For this review, take the finished solid that the model builds, in its own axes (mm). A direction names the side the tool comes from. Coordinates: 2 decimals unless noted, no trailing zeros. Write each loop counter-clockwise with the first axis right and the second up, starting at its lowest first coordinate (ties: lowest second). Pieces come first, ordered by that corner, then holes. Notation, with made-up numbers: M 0,76.25 L 5,76.25 A15 ccw 5,94.25 Z; hole C 18.5,22.5 d2. An arc over 180 degrees is marked long. One line per question, with ' | ' between items.
from build123d import *

# Parameters (mm, degrees)
F0_R     = 11.5
F0_R_2   = 8.5
F1_DEPTH = 3
F0_R_3   = 6
F2_DEPTH = 14
F3_SIZE  = 1


with BuildPart() as f1:
    # F0 (on Front) → F1 (new body)
    with BuildSketch(Plane.XZ):
        Circle(F0_R)
        Circle(F0_R_2, mode=Mode.SUBTRACT)
    extrude(amount=F1_DEPTH)

    # F0 (on Front) → F2 (join)
    with BuildSketch(Plane.XZ):
        Circle(F0_R_2)
        Circle(F0_R_3, mode=Mode.SUBTRACT)
    extrude(amount=F2_DEPTH)

    # F3
    f3_edges = [f1.edges().sort_by_distance(p)[0] for p in [
        (-8.5, -14, 0),
        (-11.5, 0, 0),
    ]]
    chamfer(f3_edges, length=F3_SIZE)


solid = f1.part
1) We need section B-B on x = 0. State the section outline as (y, z) points, then the cut area to 3 significant figures.
Responses:
outline: M -14,-7.5 L -13,-8.5 L -3,-8.5 L -3,-11.5 L -1,-11.5 L 0,-10.5 L 0,-6 L -14,-6 Z; M -14,6 L 0,6 L 0,10.5 L -1,11.5 L -3,11.5 L -3,8.5 L -13,8.5 L -14,7.5 Z | area: 86.0 mm^2
2) Machinability: for faces 1 (the flat face through (2, -14, 6)), 2 (the cylindrical face through (4.57, -7.93, 7.167)), which of the approach directions +Z, -Z, +X, -X, +Y, -Y give a long, thin tool a straight path to every point of the face, cutting with its end or side? Answer none if there is none.
Responses:
face 1: +Z, -Z, +X, -X, -Y | face 2: -Y
3) Insertion check: pin 1 Ø8 at (x, y) = (-1, -2) entering from +Z; pin 2 Ø5 at (x, y) = (2, -5) entering from -Z; pin 3 Ø1 at (x, y) = (2.5, -6.5) entering from -Z; pin 4 Ø2 at (x, y) = (0, -8.5) entering from +Z. Each pin has a flat end and moves straight along its axis. Give the tip position at first contact, or say it passes through.
Responses:
pin 1: z = 11.5 | pin 2: z = -11.49 | pin 3: z = -8.26 | pin 4: z = 8.5
4) The part is to be moulded in two halves that separate along X. For faces 3 (the cylindrical face through (-6, -7, 0)), 4 (the cylindrical face through (-1.5, -2, 11.4)), 5 (the flat face through (5, 0, -5)), say which applies: +X half, -X half, draft (parallel to the pull), parting line (faces both ways), or undercut.
Responses:
face 3: undercut | face 4: parting line | face 5: draft
5) We need section A-A on z = 0. State the section outline as (x, y) points.
Responses:
outline: M -11.5,-3 L -8.5,-3 L -8.5,-13 L -7.5,-14 L -6,-14 L -6,0 L -10.5,0 L -11.5,-1 Z; M 6,-14 L 7.5,-14 L 8.5,-13 L 8.5,-3 L 11.5,-3 L 11.5,-1 L 10.5,0 L 6,0 Z
6) To check wall thickness, follow line 1 along Z through (x, y) = (0, -10.5); line 2 along X through (y, z) = (-8.25, -3); line 3 along Y through (x, z) = (2.75, 8.5). State the ranges of each line that lie inside material, in increasing order. Write a range as [from, to].
Responses:
line 1: [-8.5, -6], [6, 8.5] | line 2: [-7.95, -5.2], [5.2, 7.95] | line 3: [-3, 0]
7) We need section C-C on y = -10.25. State the section outline as (x, z) points.
Responses:
outline: C 0,0 d17; hole C 0,0 d12
